Source: CAD feature listing. Evaluate the final solid. Frame: model axes, mm. Give positions to 0.01 mm unless a question says otherwise; leave off trailing zeros. Write each loop counter-clockwise with the first axis right and the second up, starting at its lowest first coordinate (ties: lowest second). Pieces come first, ordered by that corner, then holes. Notation, with made-up numbers: (-34, 24) -> (19, 24) arc R11 ccw to (19, 39) -> close; hole circle Ø6 at (-27, -7.5). An arc over 180 degrees is marked (long way). Answer as a JSON object with one key per item and string values. Group by question number.
Item 1: Section query A-A on x = -20. Return the cut outline in (y, z), plus the area to 3 significant figures.
Item 2: First-contact query: pin 1 Ø10.5 at (x, y) = (20, 0) entering from +Z. Flat tip, straight axial feed; report the tip coordinate or a pass-through.
Item 3: Ray query, probe 1 along Y at (x, z) = (-20, 1.05); probe 2 along Y at (x, z) = (-23.5, 0.9); probe 3 along X at (y, z) = (36.5, 1.75). Return the intervals inside material, ascending. Write a range as from..to.
Item 4: Section query B-B on z = 1.4. Return the cut outline in (x, y), plus the area to 3 significant figures.
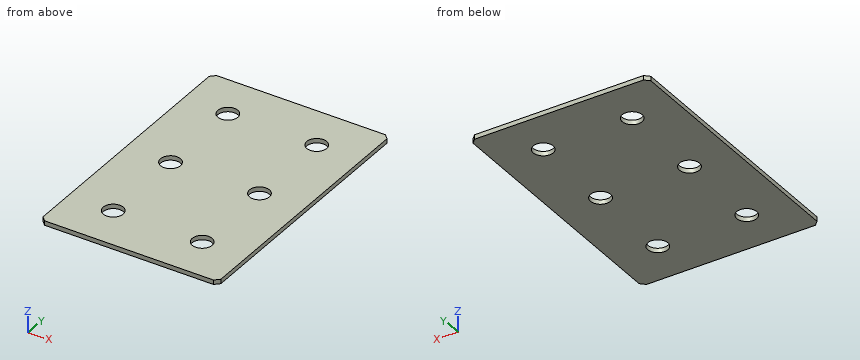
from build123d import *

# Parameters (mm, degrees)
SKETCH_1_W        = 80
SKETCH_1_H        = 120
EXTRUDE_1_DEPTH   = 2
CHAMFER_1_SIZE    = 2
HOLE_WIZARD_M81_D = 9


with BuildPart() as part:
    # Эскиз1 → Бобышка-Вытянуть1 (new body)
    with BuildSketch(Plane.XY):
        Rectangle(SKETCH_1_W, SKETCH_1_H)
    extrude(amount=EXTRUDE_1_DEPTH)

    # Фаска1
    chamfer_1_edges = [part.edges().sort_by_distance(p)[0] for p in [
        (40, -60, 1),
        (-40, -60, 1),
        (-40, 60, 1),
        (40, 60, 1),
    ]]
    chamfer(chamfer_1_edges, length=CHAMFER_1_SIZE)

    # Отверстие с зазором M81 (through all)
    with Locations(Plane.XY.offset(2)):
        with Locations((-20, 40), (20, 40), (20, 0), (-20, 0), (-20, -40), (20, -40)):
            Hole(HOLE_WIZARD_M81_D / 2)


solid = part.part
Worked answers:
{
 "1": {"outline": "(-60, 0) -> (-44.5, 0) -> (-44.5, 2) -> (-60, 2) -> close; (-35.5, 0) -> (-4.5, 0) -> (-4.5, 2) -> (-35.5, 2) -> close; (4.5, 0) -> (35.5, 0) -> (35.5, 2) -> (4.5, 2) -> close; (44.5, 0) -> (60, 0) -> (60, 2) -> (44.5, 2) -> close", "area": "186 mm^2"},
 "2": {"pin 1": "z = 2"},
 "3": {"probe 1": "-60..-44.5, -35.5..-4.5, 4.5..35.5, 44.5..60", "probe 2": "-60..-42.83, -37.17..-2.83, 2.83..37.17, 42.83..60", "probe 3": "-40..-22.83, -17.17..17.17, 22.83..40"},
 "4": {"outline": "(-40, -58) -> (-38, -60) -> (38, -60) -> (40, -58) -> (40, 58) -> (38, 60) -> (-38, 60) -> (-40, 58) -> close; hole circle Ø9 at (-20, -40); hole circle Ø9 at (-20, 0); hole circle Ø9 at (-20, 40); hole circle Ø9 at (20, -40); hole circle Ø9 at (20, 0); hole circle Ø9 at (20, 40)", "area": "9,210 mm^2"}
}
